from build123d import *

# Parameters (mm, degrees)
SKETCH061_W        = 11.8
SKETCH061_H        = 25.8
SKETCH061_W_2      = 9.8
SKETCH061_H_2      = 23.8
PAD031_DEPTH       = 15
SKETCH062_W        = 15
SKETCH062_H        = 30.5
SKETCH062_W_2      = 9.8
SKETCH062_H_2      = 23.8
PAD032_DEPTH       = 1
SKETCH063_W        = 15
SKETCH063_H        = 30.5
SKETCH063_W_2      = 13
SKETCH063_H_2      = 28.5
PAD033_DEPTH       = 15
POCKET007016_DEPTH = 30.501
SKETCH081_R        = 0.75
PAD042_DEPTH       = 7.5
SKETCH065_W        = 15.029142
SKETCH065_H        = 29.5
PAD034_DEPTH       = 1
SKETCH066_W        = 13.8
SKETCH066_H        = 5
POCKET007017_DEPTH = 3


with BuildPart() as part:
    # Sketch061 → Pad031 (new body)
    with BuildSketch(Plane.XY):
        with Locations((-57.65, -16.5)):
            Rectangle(SKETCH061_W, SKETCH061_H)
        with Locations((-57.65, -16.5)):
            Rectangle(SKETCH061_W_2, SKETCH061_H_2, mode=Mode.SUBTRACT)
    extrude(amount=PAD031_DEPTH)

    # Sketch062 → Pad032 (join)
    with BuildSketch(Plane.XY):
        with Locations((-57.65, -16.25)):
            Rectangle(SKETCH062_W, SKETCH062_H)
        with Locations((-57.65, -16.5)):
            Rectangle(SKETCH062_W_2, SKETCH062_H_2, mode=Mode.SUBTRACT)
    extrude(amount=-PAD032_DEPTH)

    # Sketch063 (on DatumPlane) → Pad033 (join)
    with BuildSketch(Plane(origin=(0, 0, 1), x_dir=(-1, 0, 0), z_dir=(0, 0, -1))):
        with Locations((57.65, -16.25)):
            Rectangle(SKETCH063_W, SKETCH063_H)
        with Locations((57.65, -16.25)):
            Rectangle(SKETCH063_W_2, SKETCH063_H_2, mode=Mode.SUBTRACT)
    extrude(amount=PAD033_DEPTH)

    # Sketch064 (on DatumPlane) → Pocket007016 (cut, through all)
    with BuildSketch(Plane(origin=(-65.15, -31.5, 1), x_dir=(1, 0, 0), z_dir=(0, -1, 0))):
        Polygon((15, -15), (0, -10.980762), (0, -15), align=None)
    extrude(amount=-POCKET007016_DEPTH, mode=Mode.SUBTRACT)

    # Sketch081 (on DatumPlane) → Pad042 (join)
    with BuildSketch(Plane.XY):
        with Locations((-57.65, -3.6)):
            Circle(SKETCH081_R)
        with Locations((-57.65, -29.4)):
            Circle(SKETCH081_R)
        with Locations((-51.75, -21.9)):
            Circle(SKETCH081_R)
        with Locations((-51.75, -11.1)):
            Circle(SKETCH081_R)
        with Locations((-63.55, -11.1)):
            Circle(SKETCH081_R)
        with Locations((-63.55, -21.9)):
            Circle(SKETCH081_R)
    extrude(amount=PAD042_DEPTH)

    # Sketch065 (on Face37 of Pocket007016) → Pad034 (join)
    with BuildSketch(Plane(origin=(-6.859413, 0, -25.599678), x_dir=(0.965926, 0, -0.258819), z_dir=(-0.258819, 0, -0.965926))):
        with Locations((-52.832285, 15.75)):
            Rectangle(SKETCH065_W, SKETCH065_H)
    extrude(amount=-PAD034_DEPTH)

    # Sketch066 (on Face36 of Pad034) → Pocket007017 (cut)
    with BuildSketch(Plane.XY.offset(7.5)):
        with Locations((-57.65, -1.1)):
            Rectangle(SKETCH066_W, SKETCH066_H)
    extrude(amount=-POCKET007017_DEPTH, mode=Mode.SUBTRACT)


with BuildPart() as part_1:
    # Body004 placement: moved
    add(part.part.moved(Location((0, -32, -16.75))))


solid = part_1.part
Design review of the part built by this model. Coordinates are the model's own, in mm. A direction names the side the tool comes from. Coordinates: 2 decimals unless noted, no trailing zeros. Write each loop counter-clockwise with the first axis right and the second up, starting at its lowest first coordinate (ties: lowest second). Pieces come first, ordered by that corner, then holes. Notation, with made-up numbers: (45.25, 43.25) - (59.25, 43.25) arc R15 ccw to (59.25, 63.25) - close; hole circle Ø9 at (-7, -14). An arc over 180 degrees is marked (long way). Use one line per item in the form item = value.
Q1. The part is to be moulded in two halves that separate along X. For faces 4 (the flat face through (-50.9, -48.2, -15.75)), 5 (the flat face through (-62.55, -49, -10)), 6 (the flat face through (-50.393, -55.099, -30.685)), say which applies: +X half, -X half, draft (parallel to the pull), parting line (faces both ways), or undercut.
Taken from the geometry:
face_4 = draft
face_5 = undercut
face_6 = -X half
Q2. Insertion check: pin 1 Ø5 at (y, z) = (-52, -8.5) entering from +X; pin 2 Ø0.8 at (x, y) = (-51, -43) entering from +Z; pin 3 Ø2 at (x, y) = (-57.5, -45.5) entering from -Z. Each pin has a flat end and moves straight along its axis. Give the tip position at first contact, or say it passes through.
Taken from the geometry:
pin_1 = -51
pin_2 = -9.25
pin_3 = -29.05
Q3. Consider section B-B (z = -10.25). Write out the cut boundary in (x, y), plus the area to 3 significant figures.
Taken from the geometry:
outline = (-63.55, -61.4) - (-58.4, -61.4) arc R0.75 ccw to (-56.9, -61.4) - (-51.75, -61.4) - (-51.75, -54.65) arc R0.75 ccw to (-51.75, -53.15) - (-51.75, -43.85) arc R0.75 ccw to (-51.75, -42.35) - (-51.75, -35.6) - (-63.55, -35.6) - (-63.55, -42.35) arc R0.75 ccw to (-63.55, -43.85) - (-63.55, -53.15) arc R0.75 ccw to (-63.55, -54.65) - close; hole (-62.55, -60.4) - (-52.75, -60.4) - (-52.75, -36.6) - (-62.55, -36.6) - close
area = 75.6 mm^2
Q4. For probe 1 along X at (y, z) = (-58.5, -24); probe 2 along X at (y, z) = (-55, -17.5); probe 3 along Y at (x, z) = (-55, -10.5), list the stretches that pass through material, from the lowest coordinate up.
Taken from the geometry:
probe_1 = -65.15 to -64.15, -51.15 to -50.15
probe_2 = -65.15 to -62.55, -52.75 to -50.15
probe_3 = -61.4 to -60.4, -36.6 to -35.6
Q5. Machinability: for faces 1 (the flat face through (-58, -33, -23)), 2 (the flat face through (-58, -36.6, -10)), 3 (the flat face through (-58, -62.5, -22)), which of the approach directions +Z, -Z, +X, -X, +Y, -Y give a long, thin tool a straight path to every point of the face, cutting with its end or side? Answer none if there is none.
Taken from the geometry:
face_1 = +Z, -Z, +X, -X, +Y
face_2 = +Z
face_3 = none
